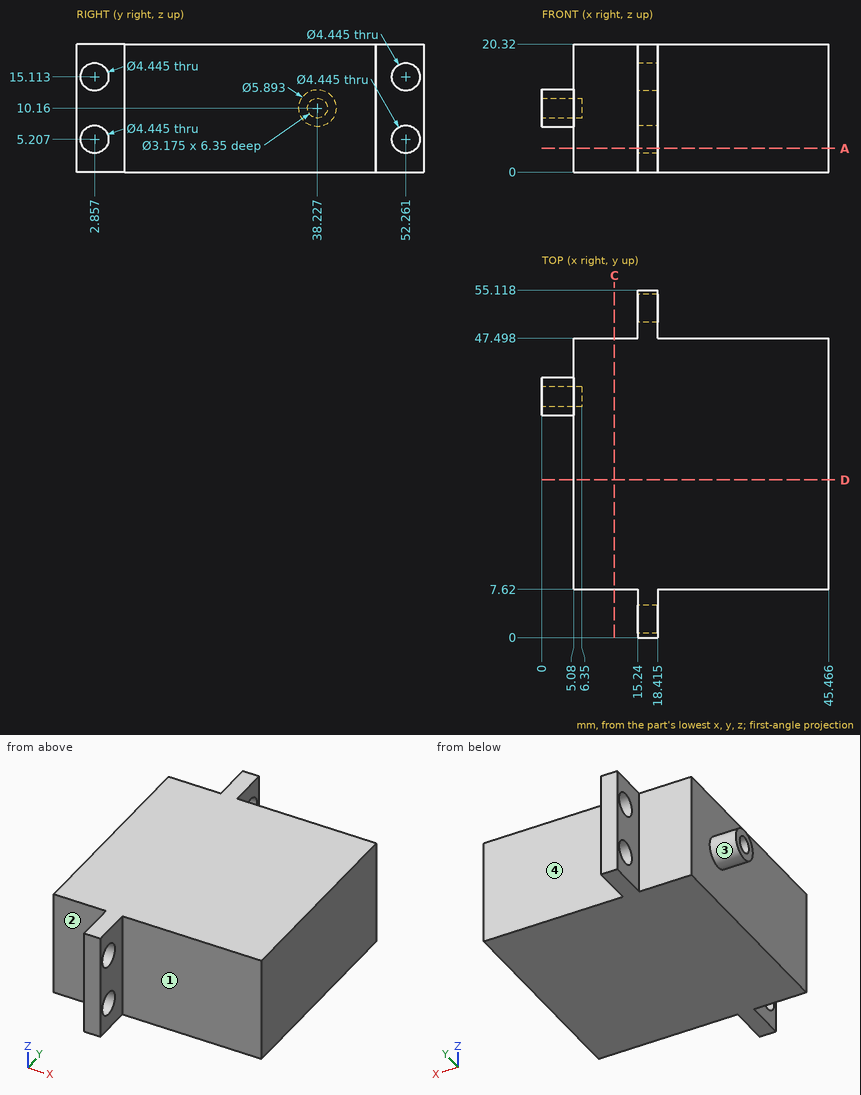
Answer from the drawing. Dimensions are ordinates in mm from the lowest x, y and z of the part. A direction names the side the tool comes from. Round coordinates to 2 decimals unless told otherwise and drop trailing zeros. Write each loop counter-clockwise with the first axis right and the second up, starting at its lowest first coordinate (ties: lowest second). Pieces come first, ordered by that corner, then holes.
1. Which of the six approach directions +Z, -Z, +X, -X, +Y, -Y give full straight-line access (tool end or side, diameter ignored) to the marked faces 1, 2, 3 and 4?
2. The part is cut by section C-C, the plane x = 11.5. Determine the outline of the cut face in (y, z).
3. The part is cut by section A-A, the plane z = 3.75. Determine the outline of the cut face in (x, y) (1 decimal), then the cut area to 3 significant figures.
4. Straight lines are drawn through the part: L1, parallel to X at y = 25, z = 8.25 (1 decimal); L2, parallel to Y at x = 39, z = 8.25; L3, parallel to X at y = 51, z = 10 (1 decimal). For each, find the intervals that lie inside material, in ascending order.
5. The part is cut by section D-D, the plane y = 25. Determine the outline of the cut face in (x, z) (1 decimal), then the cut area to 3 significant figures.
6. Given pin 1 Ø10 at (x, z) = (32, 9) entering from +Y; pin 2 Ø2.5 at (y, z) = (52.26, 15.11) entering from +X; pin 3 Ø5 at (y, z) = (2.86, 15.11) entering from +X (1 decimal); pin 4 Ø6 at (y, z) = (30.5, 9) entering from -X, each flat-ended and moving along its own axis, determine where each tip first touches the part or whether it passes through.
Values:
1. face 1: +Z, -Z, +X, -Y
1. face 2: +Z, -Z, -X, -Y
1. face 3: -X
1. face 4: +Z, -Z, +X, +Y
2. outline: (7.62, 0) - (47.5, 0) - (47.5, 20.32) - (7.62, 20.32) - close
3. outline: (5.1, 7.6) - (15.2, 7.6) - (15.2, 4.5) - (18.4, 4.5) - (18.4, 7.6) - (45.5, 7.6) - (45.5, 47.5) - (18.4, 47.5) - (18.4, 50.6) - (15.2, 50.6) - (15.2, 47.5) - (5.1, 47.5) - close; (15.2, 0) - (18.4, 0) - (18.4, 1.2) - (15.2, 1.2) - close; (15.2, 53.9) - (18.4, 53.9) - (18.4, 55.1) - (15.2, 55.1) - close
3. area: 1,640 mm2
4. L1: x = 5.1 to 45.5
4. L2: y = 7.62 to 47.5
4. L3: x = 15.2 to 18.4
5. outline: (5.1, 0) - (45.5, 0) - (45.5, 20.3) - (5.1, 20.3) - close
5. area: 821 mm2
6. pin 1: stops at y = 47.5
6. pin 2: passes through
6. pin 3: stops at x = 18.4
6. pin 4: stops at x = 5.08
